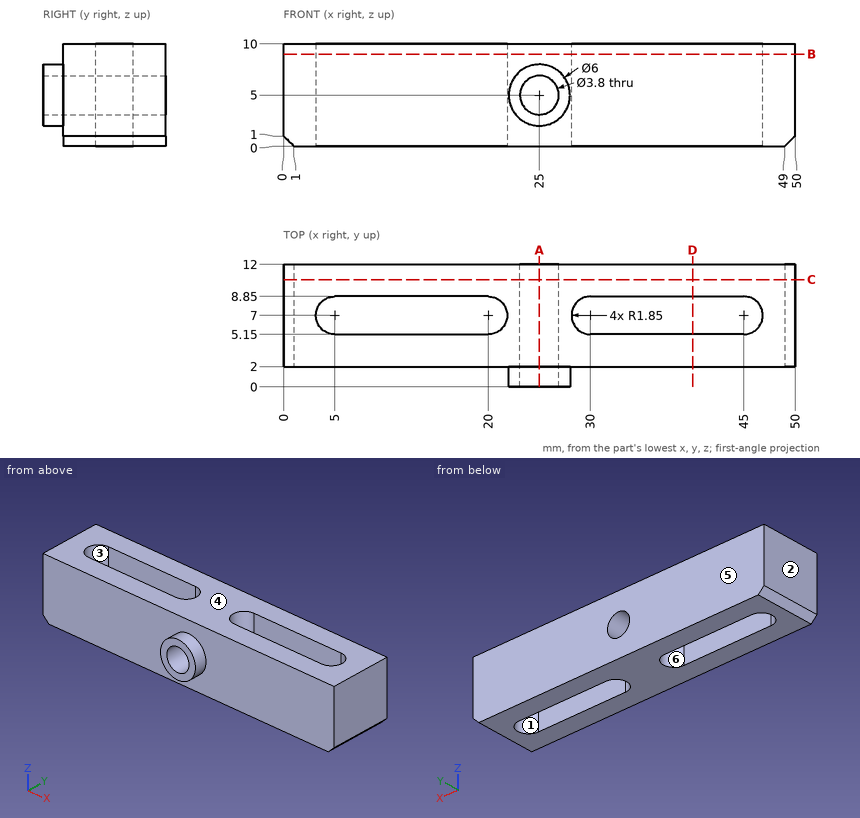
Design review of the part shown in the three views and the two pictorial views. Dimensions are in mm from the part's minimum x, y and z. A direction names the side the tool comes from. Give positions to 0.01 mm unless a question says otherwise; leave off trailing zeros. Loops run counter-clockwise (first coordinate to the right, second up) from the corner with the lowest first, then second, coordinate; pieces in that order, holes last. Notation, with made-up numbers: M -19,77 L 39,77 A32 ccw 39,104 Z; hole C -15,-10 d5. An arc over 180 degrees is marked long. Answer as a JSON object with one key per item and string values. Group by question number.
Q1. Add section C-C on y = 10.5. Give the boundary of the cut face in (x, z).
Q2. Add section B-B on z = 9. Give the boundary of the cut face in (x, y), and give its area (3 significant figures).
Q3. Mouldability with a two-part tool opening along Y and no side actions: class the marked faces 3, 4, 5 and 6 as +Y half, -Y half, draft (parallel to the pull), parting line (faces both ways), or undercut.
Q4. Tool access review of the marked faces 1 and 2: name each direction out of +Z, -Z, +X, -X, +Y, -Y from which nothing blocks a thin tool from reaching the whole face with its end or side.
Q5. For probe 1 along Y at (x, z) = (14.5, 7); probe 2 along Z at (x, y) = (25, 6.5), list the stretches that pass through material, from the lowest coordinate up. Write a range as [from, to].
Q6. Insertion check: P1, Ø2, axis at x = 37.5, z = 8.5, coming from the -Y side. The pin has a flat end and moves straight along its axis. Give the tip position at first contact, or say it passes through.
Q7. Add section D-D on x = 40. Give the boundary of the cut face in (y, z), and give its area (3 significant figures).
Q8. Add section A-A on x = 25. Give the boundary of the cut face in (y, z).
Checked values:
{
 "1": {"outline": "M 0,1 L 1,0 L 49,0 L 50,1 L 50,10 L 0,10 Z; hole C 25,5 d3.8"},
 "2": {"outline": "M 0,2 L 50,2 L 50,12 L 0,12 Z; hole M 5,5.15 L 20,5.15 A1.85 ccw 20,8.85 L 5,8.85 A1.85 ccw Z; hole M 30,5.15 L 45,5.15 A1.85 ccw 45,8.85 L 30,8.85 A1.85 ccw Z", "area": "367 mm²"},
 "3": {"face 3": "undercut", "face 4": "draft", "face 5": "+Y half", "face 6": "undercut"},
 "4": {"face 1": "+Z, -Z", "face 2": "+Z, -Z, -X, +Y, -Y"},
 "5": {"probe 1": "[2, 5.15], [8.85, 12]", "probe 2": "[0, 3.1], [6.9, 10]"},
 "6": {"P1": "y = 2"},
 "7": {"outline": "M 2,0 L 5.15,0 L 5.15,10 L 2,10 Z; M 8.85,0 L 12,0 L 12,10 L 8.85,10 Z", "area": "63.0 mm²"},
 "8": {"outline": "M 0,2 L 2,2 L 2,0 L 12,0 L 12,3.1 L 0,3.1 Z; M 0,6.9 L 12,6.9 L 12,10 L 2,10 L 2,8 L 0,8 Z"}
}
